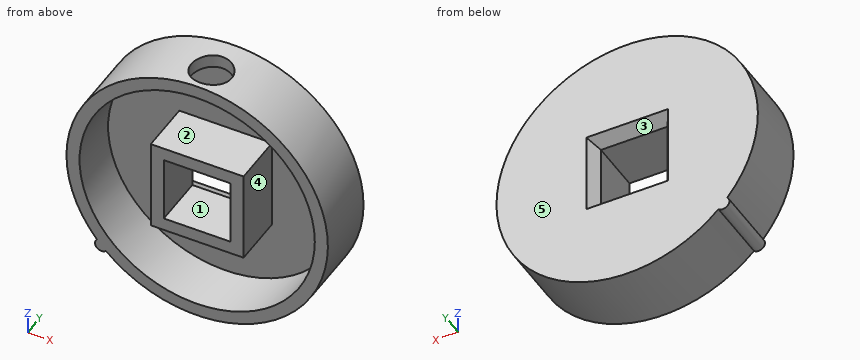
```python
from build123d import *

# Parameters (mm, degrees)
SKETCH1_R             = 20
BOSS_EXTRUDE1_DEPTH   = 10
SKETCH2_W             = 10.2
SKETCH2_H             = 10.2
CUT_EXTRUDE2_DEPTH    = 11
SHELL3_T              = -2
SKETCH3_R             = 3.1
CUT_EXTRUDE3_DEPTH    = 13.9
BOSS_EXTRUDE2_DEPTH   = 10
CHAMFER1_SIZE         = 2
CHAMFER1_SIZE2        = 1.154700538
CHAMFER1_PART_2_SIZE  = 2
CHAMFER1_PART_2_SIZE2 = 1.154700538
CHAMFER1_PART_3_SIZE  = 2
CHAMFER1_PART_3_SIZE2 = 1.154700538
CHAMFER1_PART_4_SIZE  = 2
CHAMFER1_PART_4_SIZE2 = 1.154700538


with BuildPart() as part:
    # Sketch1 → Boss-Extrude1 (new body)
    with BuildSketch(Plane(origin=(0, 0, 0), x_dir=(1, 0, 0), z_dir=(0, 1, 0))):
        Circle(SKETCH1_R)
    extrude(amount=BOSS_EXTRUDE1_DEPTH)

    # Sketch2 → Cut-Extrude2 (cut, through all)
    with BuildSketch(Plane.XZ):
        Rectangle(SKETCH2_W, SKETCH2_H)
    extrude(amount=-CUT_EXTRUDE2_DEPTH, mode=Mode.SUBTRACT)

    # Shell3
    shell3_openings = [part.faces().sort_by_distance(p)[0] for p in [
        (0, 0, 0),
    ]]
    offset(amount=SHELL3_T, openings=shell3_openings, kind=Kind.INTERSECTION)

    # Sketch3 → Cut-Extrude3 (cut, through all)
    with BuildSketch(Plane.XY.offset(7.1)):
        with Locations((0, 4)):
            Circle(SKETCH3_R)
    extrude(amount=CUT_EXTRUDE3_DEPTH, mode=Mode.SUBTRACT)

    # Sketch4 → Boss-Extrude2 (add)
    with BuildSketch(Plane(origin=(0, 10, 0), x_dir=(1, 0, 0), z_dir=(0, 1, 0))):
        with BuildLine():
            Line((-13.960317173, 14.321646009), (-15.320888862, 12.855752194))
            ThreePointArc((-15.320888862, 12.855752194), (-15.373549926, 14.268984946), (-13.960317173, 14.321646009))
        make_face()
    extrude(amount=-BOSS_EXTRUDE2_DEPTH)

    # Chamfer1
    chamfer1_edges = [part.edges().sort_by_distance(p)[0] for p in [
        (5.1, 10, 0),
    ]]
    chamfer1_side = [part.faces().sort_by_distance(p)[0] for p in [
        (5.1, 5, 0),
    ]]
    chamfer(chamfer1_edges, length=CHAMFER1_SIZE, length2=CHAMFER1_SIZE2, reference=chamfer1_side[0])

    # Chamfer1 part 2
    chamfer1_part_2_edges = [part.edges().sort_by_distance(p)[0] for p in [
        (0, 10, -5.1),
    ]]
    chamfer1_part_2_side = [part.faces().sort_by_distance(p)[0] for p in [
        (0, 5, -5.1),
    ]]
    chamfer(chamfer1_part_2_edges, length=CHAMFER1_PART_2_SIZE, length2=CHAMFER1_PART_2_SIZE2, reference=chamfer1_part_2_side[0])

    # Chamfer1 part 3
    chamfer1_part_3_edges = [part.edges().sort_by_distance(p)[0] for p in [
        (-5.1, 10, 0),
    ]]
    chamfer1_part_3_side = [part.faces().sort_by_distance(p)[0] for p in [
        (-5.1, 5, 0),
    ]]
    chamfer(chamfer1_part_3_edges, length=CHAMFER1_PART_3_SIZE, length2=CHAMFER1_PART_3_SIZE2, reference=chamfer1_part_3_side[0])

    # Chamfer1 part 4
    chamfer1_part_4_edges = [part.edges().sort_by_distance(p)[0] for p in [
        (0, 10, 5.1),
    ]]
    chamfer1_part_4_side = [part.faces().sort_by_distance(p)[0] for p in [
        (0, 5, 5.1),
    ]]
    chamfer(chamfer1_part_4_edges, length=CHAMFER1_PART_4_SIZE, length2=CHAMFER1_PART_4_SIZE2, reference=chamfer1_part_4_side[0])


solid = part.part
```
Geometry: final body of the model. Coordinates: model frame, mm. Face numbers are marked on the shaded views. A direction names the side the tool comes from. Round coordinates to 2 decimals unless told otherwise and drop trailing zeros. Write each loop counter-clockwise with the first axis right and the second up, starting at its lowest first coordinate (ties: lowest second). Pieces come first, ordered by that corner, then holes. Notation, with made-up numbers: (22, 28.25) -> (73, 28.25) arc R18 ccw to (73, 49.25) -> close; hole circle Ø3 at (62, 57). An arc over 180 degrees is marked (long way). Use CSV: the item, a comma, the result in double quotes. Start each with the question number.
Q1. Pull-direction query (Z, two-part tool) for the marked faces 4 and 5; classes: pulls with the +Z half, pulls with the -Z half, needs draft (parallel to the pull), parting line crosses it, or undercut.
Q2. Section D-D (z = 8). Return loops of the section in (x, y), plus the area to 3 significant figures.
Q3. Section C-C (x = -1.5). Return loops of the section in (y, z), plus the area to 3 significant figures.
Q4. Section B-B (y = 2.75). Return loops of the section in (x, z).
Q5. Reachability of the marked faces 1, 2 and 3 from +Z, -Z, +X, -X, +Y, -Y: full face, straight path, thin tool, end or side. Return the list, or none.
Q6. Line query: L1, parallel to X at y = 7.25, z = -0.5; L2, parallel to Z at x = 0, y = 3; L3, parallel to X at y = 2.75, z = 3. Output: solid intervals per line, ascending.
Q7. First-contact query: pin 1 Ø1.5 at (x, y) = (3, 3.5) entering from +Z; pin 2 Ø1.5 at (x, y) = (9, 3.5) entering from -Z; pin 3 Ø2.5 at (x, y) = (0.5, 3.5) entering from +Z. Flat tips, straight axial feed; report the tip coordinate or a pass-through.
Q8. Section A-A (z = 0). Return loops of the section in (x, y).
Result sheet:
1,face 4,"undercut"
1,face 5,"needs draft"
2,outline,"(-18.33, 0) -> (-16.12, 0) -> (-16.12, 8) -> (16.12, 8) -> (16.12, 0) -> (18.33, 0) -> (18.33, 10) -> (-18.33, 10) -> close"
2,area,"109 mm²"
3,outline,"(0, -19.94) -> (10, -19.94) -> (10, -6.25) -> (8, -5.1) -> (0, -5.1) -> (0, -7.1) -> (8, -7.1) -> (8, -17.94) -> (0, -17.94) -> close; (0, 5.1) -> (8, 5.1) -> (10, 6.25) -> (10, 19.94) -> (6.71, 19.94) -> (6.71, 17.94) -> (8, 17.94) -> (8, 7.1) -> (0, 7.1) -> close; (0, 17.94) -> (1.29, 17.94) -> (1.29, 19.94) -> (0, 19.94) -> close"
3,area,"110 mm²"
4,outline,"(-15.32, -12.86) arc R1 ccw to (-13.96, -14.32) arc R20 ccw (long way) to (2.84, 19.8) -> (2.84, 17.78) arc R18 cw (long way) to (-2.84, 17.78) -> (-2.84, 19.8) arc R20 ccw to start; (-7.1, -7.1) -> (7.1, -7.1) -> (7.1, 7.1) -> (-7.1, 7.1) -> close; hole (-5.1, -5.1) -> (5.1, -5.1) -> (5.1, 5.1) -> (-5.1, 5.1) -> close"
5,face 1,"+Y, -Y"
5,face 2,"-Y"
5,face 3,"+Y"
6,L1,"-19.99 to -17.99, -7.1 to -5.1, 5.1 to 7.1, 17.99 to 19.99"
6,L2,"-20 to -18, -7.1 to -5.1, 5.1 to 7.1"
6,L3,"-19.77 to -17.75, -7.1 to -5.1, 5.1 to 7.1, 17.75 to 19.77"
7,pin 1,"z = 19.8"
7,pin 2,"z = -18.22"
7,pin 3,"z = 7.1"
8,outline,"(-20, 0) -> (-18, 0) -> (-18, 8) -> (-7.1, 8) -> (-7.1, 0) -> (-5.1, 0) -> (-5.1, 8) -> (-6.25, 10) -> (-20, 10) -> close; (5.1, 0) -> (7.1, 0) -> (7.1, 8) -> (18, 8) -> (18, 0) -> (20, 0) -> (20, 10) -> (6.25, 10) -> (5.1, 8) -> close"
